Part model, mm, in its own coordinate system. A direction names the side the tool comes from. Round coordinates to 2 decimals unless told otherwise and drop trailing zeros. Write each loop counter-clockwise with the first axis right and the second up, starting at its lowest first coordinate (ties: lowest second). Pieces come first, ordered by that corner, then holes. Notation, with made-up numbers: (76.25, -2.5) -> (127.25, -2.5) arc R23 ccw to (127.25, 26.5) -> close; hole circle Ø10 at (-23.75, 64). An arc over 180 degrees is marked (long way). Return JSON: item names as keys, results as strings. Group by question number.
(1) Saw through at A-A (z = 0). List the corners of the cut face in (x, y).
(2) Saw through at B-B (y = 173). List the corners of the cut face in (x, z), plus the area to 3 significant figures.
(3) Drill centre lines: L1, parallel to X at y = 62.5, z = 0; L2, parallel to X at y = 72.5, z = 9.5; L3, parallel to X at y = 298, z = -171. Where is each one in solid material? Low to high. Write a range as from..to.
(4) Drop flat-ended pins along their axis: pin 1 Ø4 at (x, y) = (-1389, -67) entering from -Z; pin 2 Ø6 at (x, z) = (-1109.5, -122.5) entering from -Y; pin 3 Ø1.5 at (x, y) = (-232.5, 73.5) entering from +Z. Give the stop position or say it passes through.
(5) Saw through at D-D (x = -150). List the corners of the cut face in (y, z).
(6) Saw through at C-C (z = 196). List the corners of the cut face in (x, y).
(7) Tool access for faces 1 (the cylindrical face through (-735.15, -249.76, 10.99)), 2 (the cylindrical face through (-1510.84, -257.96, 236.55)): list every direction of +Z, -Z, +X, -X, +Y, -Y with a clear straight run to the whole face (end or side of a thin tool).
from build123d import *

# Parameters (mm, degrees)
SKETCH3_R               = 30
CUT_EXTRUDE1_DEPTH      = 351
CUT_EXTRUDE1_DEPTH_BACK = 351


with BuildPart() as part:
    # Sketch2 → Revolve1 (revolve)
    with BuildSketch(Plane.XY):
        Polygon((0, 0), (0, 250), (-1450, 250), (-1450, 350), (-1570, 350), (-1570, 0), align=None)
    revolve(axis=Axis((-1570, 0, 0), (1, 0, 0)))

    # Sketch3 → Cut-Extrude1 (cut, two sides)
    with BuildSketch(Plane(origin=(0, 0, 0), x_dir=(1, 0, 0), z_dir=(0, 1, 0))) as cut_extrude1_sk:
        with Locations((-150, 0)):
            Circle(SKETCH3_R)
    extrude(amount=CUT_EXTRUDE1_DEPTH, mode=Mode.SUBTRACT)
    extrude(cut_extrude1_sk.sketch, amount=-CUT_EXTRUDE1_DEPTH_BACK, mode=Mode.SUBTRACT)


solid = part.part
Computed values:
{
 "1": {"outline": "(-1570, -350) -> (-1450, -350) -> (-1450, -250) -> (-180, -250) -> (-180, 250) -> (-1450, 250) -> (-1450, 350) -> (-1570, 350) -> close; (-120, -250) -> (0, -250) -> (0, 250) -> (-120, 250) -> close"},
 "2": {"outline": "(-1570, -304.25) -> (-1450, -304.25) -> (-1450, -180.47) -> (0, -180.47) -> (0, 180.47) -> (-1450, 180.47) -> (-1450, 304.25) -> (-1570, 304.25) -> close; hole circle Ø60 at (-150, 0)", "area": "594,000 mm2"},
 "3": {"L1": "-1570..-180, -120..0", "L2": "-1570..-178.46, -121.54..0", "L3": "-1570..-1450"},
 "4": {"pin 1": "z = -241.4", "pin 2": "y = -219.59", "pin 3": "z = 239.18"},
 "5": {"outline": "(-248.19, -30) arc R250 ccw to (248.19, -30) -> close; (-248.19, 30) -> (248.19, 30) arc R250 ccw to start"},
 "6": {"outline": "(-1570, -289.97) -> (-1450, -289.97) -> (-1450, -155.19) -> (0, -155.19) -> (0, 155.19) -> (-1450, 155.19) -> (-1450, 289.97) -> (-1570, 289.97) -> close"},
 "7": {"face 1": "+X", "face 2": "+X, -X"}
}
